Build history of the part. All positions in model axes, mm. A direction names the side the tool comes from. Round coordinates to 2 decimals unless told otherwise and drop trailing zeros. Order: outer loops, then holes, each group sorted by start corner. A loop starts at its lowest first (then second) coordinate and runs counter-clockwise, first axis right, second up. Notation, with made-up numbers: (-30.5, 70.25) -> (12.5, 70.25) arc R17 cw to (12.5, 89.25) -> close; hole circle Ø9 at (75.25, 84). An arc over 180 degrees is marked (long way). Use a Markdown table: item, result. Add a question column.
Item 1: Slice it at C-C, the plane y = 13.5. Give the cut face in (x, z) (3 decimals), plus the area to 3 significant figures.
Item 2: Slice it at A-A, the plane x = -21.5. Give the cut face in (y, z) (3 decimals), plus the area to 3 significant figures.
Item 3: Pin check, flat tips, straight feed: pin 1 (6 mm diameter, centred on x = -15, z = -31.5, fed in from -Y); pin 2 (4 mm diameter, centred on x = -30, y = 12.5, fed in from -Z); pin 3 (2 mm diameter, centred on x = -7.747, z = -19.05, fed in from -Y) (3 decimals). Stop position of each tip, or through.
Item 4: 3-axis set-ups, long thin cutter, end or side, ignore diameter. For faces 1 (the face through (-18, 3.175, -19)), 2 (the face through (0, 9, -19)), 3 (the face through (-8.7, 1.57, -20.55)), 4 (the face through (-1.57, 6.99, -10.31)): which of +Z, -Z, +X, -X, +Y, -Y reach the whole face in a straight line?
Item 5: Slice it at B-B, the plane z = -19.05. Give the cut face in (x, y) (3 decimals), plus the area to 3 significant figures.
Item 6: Slice it at D-D, the plane z = -4. Give the cut face in (x, y) (3 decimals), plus the area to 3 significant figures.
Item 7: Probe L1, parallel to X at y = 1.65, z = -19.05 (3 decimals); L2, parallel to Y at x = -11, z = -7 (3 decimals); L3, parallel to X at y = 4.5, z = -12 (3 decimals). List the from-to ranges inside material, lowest first.
Item 8: Two-plate mould, pull along Z, no slides. Class faces 5 (the face through (-26.312, 1.565, -20.813)), 6 (the face through (-18, 18, 0)), 7 (the face through (-18, 19.05, -19)), 8 (the face through (-18, 18, -38.1)): released by +Z, released by -Z, zero draft, split by the parting line, or undercut.
from build123d import *

# Parameters (mm, degrees)
BOSS_EXTRUDE1_DEPTH = 38.1
SKETCH2_R           = 1.778
CUT_EXTRUDE1_DEPTH  = 15.24
SKETCH4_W           = 18.034
SKETCH4_H           = 3.175
BOSS_EXTRUDE2_DEPTH = 38.1
SKETCH3_R           = 1.778
CUT_EXTRUDE2_DEPTH  = 15.24


with BuildPart() as part:
    # Sketch1 → Boss-Extrude1 (new body)
    with BuildSketch(Plane.XY):
        Polygon((0, 0), (0, 19.05), (-35.814, 19.05), (-35.814, 0), (-21.209, 0), (-21.209, 3.175), (-32.639, 3.175), (-32.639, 15.875), (-3.175, 15.875), (-3.175, 0), align=None)
    extrude(amount=-BOSS_EXTRUDE1_DEPTH)

    # Sketch2 → Cut-Extrude1 (cut)
    with BuildSketch(Plane(origin=(0, 0, 0), x_dir=(0, 0, -1), z_dir=(1, 0, 0))):
        with Locations((12.0859042, 6.91388)):
            Circle(SKETCH2_R)
        with Locations((26.0140958, 6.91388)):
            Circle(SKETCH2_R)
    extrude(amount=-CUT_EXTRUDE1_DEPTH, mode=Mode.SUBTRACT)

    # Sketch4 → Boss-Extrude2 (add)
    with BuildSketch(Plane.XY):
        with Locations((-12.192, 1.5875)):
            Rectangle(SKETCH4_W, SKETCH4_H)
    extrude(amount=-BOSS_EXTRUDE2_DEPTH)

    # Sketch3 → Cut-Extrude2 (cut)
    with BuildSketch(Plane(origin=(0, 0, 0), x_dir=(-1, 0, 0), z_dir=(0, -1, 0))):
        with Locations((26.543, 19.05)):
            Circle(SKETCH3_R)
        with Locations((7.747, 19.05)):
            Circle(SKETCH3_R)
    extrude(amount=-CUT_EXTRUDE2_DEPTH, mode=Mode.SUBTRACT)


solid = part.part
Check sheet entries:
| question | item | result |
|---|---|---|
| 1 | outline | (-35.814, -38.1) -> (-32.639, -38.1) -> (-32.639, 0) -> (-35.814, 0) -> close; (-3.175, -38.1) -> (0, -38.1) -> (0, 0) -> (-3.175, 0) -> close |
| 1 | area | 242 mm2 |
| 2 | outline | (0, -38.1) -> (3.175, -38.1) -> (3.175, 0) -> (0, 0) -> close; (15.875, -38.1) -> (19.05, -38.1) -> (19.05, 0) -> (15.875, 0) -> close |
| 2 | area | 242 mm2 |
| 3 | pin 1 | y = 0 |
| 3 | pin 2 | through |
| 3 | pin 3 | y = 15.875 |
| 4 | face 1 | +Z, -Z |
| 4 | face 2 | +Z, -Z, +X, +Y, -Y |
| 4 | face 3 | -Y |
| 4 | face 4 | +X |
| 5 | outline | (-35.814, 0) -> (-28.321, 0) -> (-28.321, 3.175) -> (-32.639, 3.175) -> (-32.639, 15.875) -> (-3.175, 15.875) -> (-3.175, 3.175) -> (-5.969, 3.175) -> (-5.969, 0) -> (0, 0) -> (0, 19.05) -> (-35.814, 19.05) -> close; (-24.765, 0) -> (-9.525, 0) -> (-9.525, 3.175) -> (-24.765, 3.175) -> close |
| 5 | area | 285 mm2 |
| 6 | outline | (-35.814, 0) -> (0, 0) -> (0, 19.05) -> (-35.814, 19.05) -> close; hole (-32.639, 3.175) -> (-3.175, 3.175) -> (-3.175, 15.875) -> (-32.639, 15.875) -> close |
| 6 | area | 308 mm2 |
| 7 | L1 | -35.814 to -28.321, -24.765 to -9.525, -5.969 to 0 |
| 7 | L2 | 0 to 3.175, 15.875 to 19.05 |
| 7 | L3 | -35.814 to -32.639, -3.175 to 0 |
| 8 | face 5 | undercut |
| 8 | face 6 | released by +Z |
| 8 | face 7 | zero draft |
| 8 | face 8 | released by -Z |
